Input: part model. Units: mm. Frame: model coordinates. A direction names the side the tool comes from. Round coordinates to 2 decimals unless told otherwise and drop trailing zeros. Loops run counter-clockwise (first coordinate to the right, second up) from the corner with the lowest first, then second, coordinate; pieces in that order, holes last. Notation, with made-up numbers: (-3.75, 63) -> (54.25, 63) arc R19 ccw to (54.25, 79) -> close; hole circle Ø3 at (83, 27.5). An arc over 180 degrees is marked (long way). Answer as a JSON object with one key per item and string values.
```python
from build123d import *

# Parameters (mm, degrees)
SKETCH2_W           = 65
SKETCH2_H           = 100
SKETCH2_R           = 1.75
SKETCH2_R_2         = 2.65
BOSS_EXTRUDE1_DEPTH = 5
SKETCH3_R           = 4.5
CUT_EXTRUDE1_DEPTH  = 2.5
FILLET1_R           = 5
CHAMFER1_SIZE       = 1.6
CUT_EXTRUDE2_DEPTH  = 60.843546018
FILLET3_R           = 5
FILLET2_R           = 2


with BuildPart() as part:
    # Sketch2 → Boss-Extrude1 (new body)
    with BuildSketch(Plane(origin=(0, 0, 0), x_dir=(1, 0, 0), z_dir=(0, 1, 0))):
        Rectangle(SKETCH2_W, SKETCH2_H)
        with Locations(Location((-27.5, 40, 0), (0, 0, 270))):
            Circle(SKETCH2_R, mode=Mode.SUBTRACT)
        with Locations(Location((-27.5, -40, 0), (0, 0, 270))):
            Circle(SKETCH2_R, mode=Mode.SUBTRACT)
        with Locations(Location((23.6525, 28.725, 0), (0, 0, 270))):
            Circle(SKETCH2_R_2, mode=Mode.SUBTRACT)
        with Locations(Location((13.65, -28.4925, 0), (0, 0, 270))):
            Circle(SKETCH2_R_2, mode=Mode.SUBTRACT)
    extrude(amount=BOSS_EXTRUDE1_DEPTH)

    # Sketch3 → Cut-Extrude1 (cut)
    with BuildSketch(Plane(origin=(0, 5, 0), x_dir=(1, 0, 0), z_dir=(0, 1, 0))):
        with Locations(Location((23.6525, 28.725, 0), (0, 0, 270))):
            Circle(SKETCH3_R)
        with Locations(Location((13.65, -28.4925, 0), (0, 0, 270))):
            Circle(SKETCH3_R)
    extrude(amount=-CUT_EXTRUDE1_DEPTH, mode=Mode.SUBTRACT)

    # Fillet1
    fillet1_edges = [part.edges().sort_by_distance(p)[0] for p in [
        (32.5, 2.5, 50),
        (-32.5, 2.5, 50),
        (-32.5, 2.5, -50),
        (32.5, 2.5, -50),
    ]]
    fillet(fillet1_edges, radius=FILLET1_R)

    # Chamfer1
    chamfer1_edges = [part.edges().sort_by_distance(p)[0] for p in [
        (-27.5, 5, -41.75),
        (-27.5, 5, 38.25),
    ]]
    chamfer(chamfer1_edges, length=CHAMFER1_SIZE)

    # Sketch4 → Cut-Extrude2 (cut, through all)
    with BuildSketch(Plane(origin=(0, 5, 0), x_dir=(1, 0, 0), z_dir=(0, 1, 0))):
        Polygon((7.5, 7.5), (7.5, -7.5), (32.5, -20), (32.5, 20), align=None)
    extrude(amount=-CUT_EXTRUDE2_DEPTH, mode=Mode.SUBTRACT)

    # Fillet3
    fillet3_edges = [part.edges().sort_by_distance(p)[0] for p in [
        (7.5, 2.5, -7.5),
        (32.5, 2.5, -20),
        (32.5, 2.5, 20),
        (7.5, 2.5, 7.5),
    ]]
    fillet(fillet3_edges, radius=FILLET3_R)

    # Fillet2
    # the kernel refuses this fillet: 2 mm, written as the material it takes off along each edge
    with BuildSketch(Plane(origin=(12.5, 5, 4.409830056), x_dir=(-0.447213595499958, 0, 0.894427190999916), z_dir=(0.894427190999916, 0, 0.447213595499958))) as fillet2_piece_1:
        with BuildLine():
            CenterArc((5 + FILLET2_R, FILLET2_R), FILLET2_R, 180, 90)
            Line((5, FILLET2_R), (5, 0))
            Line((5, 0), (5 + FILLET2_R, 0))
        make_face()
    revolve(axis=Axis((12.5, 5, 4.409830056), (0, -1, 0)), revolution_arc=63.434948823, mode=Mode.SUBTRACT)
    with BuildSketch(Plane(origin=(12.5, 5, -4.409830056), x_dir=(-1, 0, 0), z_dir=(0, 0, 1))) as fillet2_piece_2:
        with BuildLine():
            CenterArc((5 + FILLET2_R, FILLET2_R), FILLET2_R, 180, 90)
            Line((5, FILLET2_R), (5, 0))
            Line((5, 0), (5 + FILLET2_R, 0))
        make_face()
    revolve(axis=Axis((12.5, 5, -4.409830056), (0, -1, 0)), revolution_arc=63.434948823, mode=Mode.SUBTRACT)
    with BuildSketch(Plane(origin=(32.5, 5, 23.090169944), x_dir=(-1, 0, 0), z_dir=(0, 0, 1)), Plane(origin=(32.5, 5, -45), x_dir=(-1, 0, 0), z_dir=(0, 0, 1))) as fillet2_piece_3:
        with BuildLine():
            CenterArc((FILLET2_R, FILLET2_R), FILLET2_R, 180, 90)
            Line((0, FILLET2_R), (0, 0))
            Line((0, 0), (FILLET2_R, 0))
        make_face()
    extrude(amount=21.909830056, mode=Mode.SUBTRACT)
    with BuildSketch(Plane(origin=(27.5, 5, 50), x_dir=(0, 0, -1), z_dir=(-1, 0, 0)), Plane(origin=(-27.5, 5, -50), x_dir=(0, 0, 1), z_dir=(1, 0, 0))) as fillet2_piece_4:
        with BuildLine():
            CenterArc((FILLET2_R, FILLET2_R), FILLET2_R, 180, 90)
            Line((0, FILLET2_R), (0, 0))
            Line((0, 0), (FILLET2_R, 0))
        make_face()
    extrude(amount=55, mode=Mode.SUBTRACT)
    with BuildSketch(Plane(origin=(-32.5, 5, 45), x_dir=(1, 0, 0), z_dir=(0, 0, -1))) as fillet2_piece_5:
        with BuildLine():
            CenterArc((FILLET2_R, FILLET2_R), FILLET2_R, 180, 90)
            Line((0, FILLET2_R), (0, 0))
            Line((0, 0), (FILLET2_R, 0))
        make_face()
    extrude(amount=90, mode=Mode.SUBTRACT)
    with BuildSketch(Plane(origin=(-27.5, 5, 45), x_dir=(-1, 0, 0), z_dir=(0, 0, -1))) as fillet2_piece_6:
        with BuildLine():
            CenterArc((5 - FILLET2_R, -FILLET2_R), FILLET2_R, 0, 90)
            Line((5, -FILLET2_R), (5, 0))
            Line((5, 0), (5 - FILLET2_R, 0))
        make_face()
    revolve(axis=Axis((-27.5, 5, 45), (0, 1, 0)), revolution_arc=90, mode=Mode.SUBTRACT)
    with BuildSketch(Plane(origin=(27.5, 5, -45), x_dir=(0, 0, -1), z_dir=(-1, 0, 0))) as fillet2_piece_7:
        with BuildLine():
            CenterArc((5 - FILLET2_R, FILLET2_R), FILLET2_R, 270, 90)
            Line((5, FILLET2_R), (5, 0))
            Line((5, 0), (5 - FILLET2_R, 0))
        make_face()
    revolve(axis=Axis((27.5, 5, -45), (0, -1, 0)), revolution_arc=90, mode=Mode.SUBTRACT)
    with BuildSketch(Plane(origin=(-27.5, 5, -45), x_dir=(0, 0, -1), z_dir=(1, 0, 0))) as fillet2_piece_8:
        with BuildLine():
            CenterArc((5 - FILLET2_R, -FILLET2_R), FILLET2_R, 0, 90)
            Line((5, -FILLET2_R), (5, 0))
            Line((5, 0), (5 - FILLET2_R, 0))
        make_face()
    revolve(axis=Axis((-27.5, 5, -45), (0, 1, 0)), revolution_arc=90, mode=Mode.SUBTRACT)
    with BuildSketch(Plane(origin=(27.5, 5, 45), x_dir=(1, 0, 0), z_dir=(0, 0, -1))) as fillet2_piece_9:
        with BuildLine():
            CenterArc((5 - FILLET2_R, FILLET2_R), FILLET2_R, 270, 90)
            Line((5, FILLET2_R), (5, 0))
            Line((5, 0), (5 - FILLET2_R, 0))
        make_face()
    revolve(axis=Axis((27.5, 5, 45), (0, -1, 0)), revolution_arc=90, mode=Mode.SUBTRACT)
    with BuildSketch(Plane(origin=(29.736067977, 5, -18.618033989), x_dir=(-0.4472135954999579, 0, -0.8944271909999159), z_dir=(-0.894427190999916, 0, 0.4472135954999579)), Plane(origin=(10.263932023, 5, 8.881966011), x_dir=(-0.4472135954999579, 0, 0.894427190999916), z_dir=(0.894427190999916, 0, 0.4472135954999579))) as fillet2_piece_10:
        with BuildLine():
            CenterArc((FILLET2_R, FILLET2_R), FILLET2_R, 180, 90)
            Line((0, FILLET2_R), (0, 0))
            Line((0, 0), (FILLET2_R, 0))
        make_face()
    extrude(amount=21.770509831, mode=Mode.SUBTRACT)
    with BuildSketch(Plane(origin=(7.5, 5, -4.409830056), x_dir=(-1, 0, 0), z_dir=(0, 0, 1))) as fillet2_piece_11:
        with BuildLine():
            CenterArc((FILLET2_R, FILLET2_R), FILLET2_R, 180, 90)
            Line((0, FILLET2_R), (0, 0))
            Line((0, 0), (FILLET2_R, 0))
        make_face()
    extrude(amount=8.819660113, mode=Mode.SUBTRACT)
    with BuildSketch(Plane(origin=(27.5, 5, 23.090169944), x_dir=(1, 0, 0), z_dir=(0, 0, 1))) as fillet2_piece_12:
        with BuildLine():
            CenterArc((5 - FILLET2_R, -FILLET2_R), FILLET2_R, 0, 90)
            Line((5, -FILLET2_R), (5, 0))
            Line((5, 0), (5 - FILLET2_R, 0))
        make_face()
    revolve(axis=Axis((27.5, 5, 23.090169944), (0, 1, 0)), revolution_arc=63.434948823, mode=Mode.SUBTRACT)
    with BuildSketch(Plane(origin=(27.5, 5, -23.090169944), x_dir=(0.44721359549995743, 0, 0.8944271909999162), z_dir=(-0.8944271909999162, 0, 0.44721359549995743))) as fillet2_piece_13:
        with BuildLine():
            CenterArc((5 - FILLET2_R, -FILLET2_R), FILLET2_R, 0, 90)
            Line((5, -FILLET2_R), (5, 0))
            Line((5, 0), (5 - FILLET2_R, 0))
        make_face()
    revolve(axis=Axis((27.5, 5, -23.090169944), (0, 1, 0)), revolution_arc=63.434948823, mode=Mode.SUBTRACT)


solid = part.part
```
1) Contact query for flat-ended pins moving along their axis: P1, Ø10, axis at x = 26, z = -29, coming from the +Y side; P2, Ø5.5, axis at x = 13.65, z = 28.49, coming from the +Y side. Output: stop coordinate, or through.
Output:
{"P1": "stops at y = 5", "P2": "stops at y = 2.5"}
2) Section B-B, the plane x = 13.65. Count the separate pieces of the cut face and the enclosed holes in it, plus the area to 3 significant figures.
Output:
{"separate pieces": "3", "enclosed holes": "0", "area": "355 mm^2"}
3) Ray query, probe 1 along X at (y, z) = (0.8, -40); probe 2 along Z at (x, y) = (13.65, 1.9) (1 decimal); probe 3 along X at (y, z) = (4.2, 30). Return the intervals inside material, ascending.
Output:
{"probe 1": "x = -32.5 to -29.25, -25.75 to 32.5", "probe 2": "z = -50 to -10.6, 10.6 to 25.8, 31.1 to 50", "probe 3": "x = -32.1 to 9.41, 17.89 to 32.1"}
4) Draft query along Z for faces 1 (the face through (0, 5, -1)), 2 (the face through (19.609, 4.399, 14.192)), 3 (the face through (31.733, 1.479, 20.429)), 4 (the face through (31, 1.52, 48.57)). Return one class per face: +Z half, -Z half, draft (parallel to the pull), parting line (faces both ways), or undercut.
Output:
{"face 1": "draft", "face 2": "undercut", "face 3": "undercut", "face 4": "+Z half"}
5) Reachability of faces 5 (the face through (26.694, 3.768, -32.042)), 6 (the face through (31.77, 1.48, -20.49)), 7 (the face through (0, 1, 50)) from +Z, -Z, +X, -X, +Y, -Y: full face, straight path, thin tool, end or side. Return the list, or none.
Output:
{"face 5": "+Y", "face 6": "+X, +Y, -Y", "face 7": "+Z, +X, -X, +Y, -Y"}
6) Section C-C, the plane z = 27.5. Output: boundary loops of the cut face in (x, y), plus the area to 3 significant figures.
Output:
{"outline": "(-32.5, 0) -> (11.19, 0) -> (11.19, 2.5) -> (9.26, 2.5) -> (9.26, 5) -> (-30.5, 5) arc R2 ccw to (-32.5, 3) -> close; (16.11, 0) -> (32.5, 0) -> (32.5, 3) arc R2 ccw to (30.5, 5) -> (18.04, 5) -> (18.04, 2.5) -> (16.11, 2.5) -> close", "area": "289 mm^2"}
7) Section A-A, the plane z = -40. Output: boundary loops of the cut face in (x, y).
Output:
{"outline": "(-32.5, 0) -> (-29.25, 0) -> (-29.25, 3.4) -> (-30.82, 4.97) arc R2 ccw to (-32.5, 3) -> close; (-25.75, 0) -> (32.5, 0) -> (32.5, 3) arc R2 ccw to (30.5, 5) -> (-24.15, 5) -> (-25.75, 3.4) -> close"}
